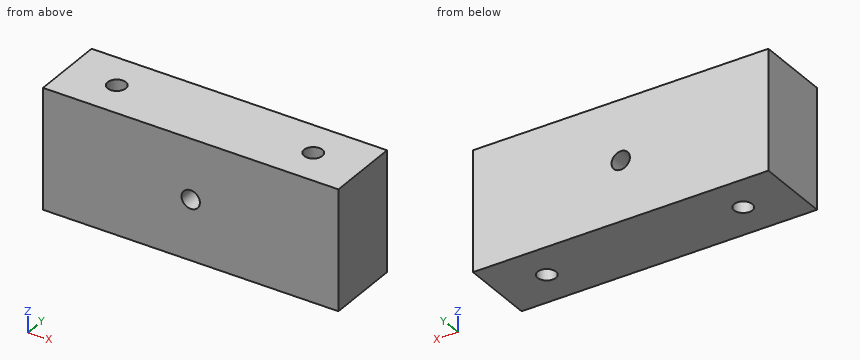
```python
from build123d import *

# Parameters (mm, degrees)
BOSS_EXTRUDE1_START     = 0.05
BOSS_EXTRUDE1_DEPTH     = 18.32
CUT_EXTRUDE1_DEPTH      = 168.935502816
CUT_EXTRUDE1_DEPTH_BACK = 168.935502816
SKETCH2_R               = 1.4
SKETCH3_R               = 1.4
CUT_EXTRUDE2_DEPTH      = 65.399803221


with BuildPart() as part:
    # Sketch1 → Boss-Extrude1 (new body)
    with BuildSketch(Plane.XY.offset(BOSS_EXTRUDE1_START)):
        Polygon((60.67170061, -154.017379901), (60.67170061, -144.167379901), (15.57170061, -144.167379901), (15.57170061, -154.017379901), (15.57170061, -155.517379901), (60.67170061, -155.517379901), align=None)
    extrude(amount=BOSS_EXTRUDE1_DEPTH)

    # Sketch2 → Cut-Extrude1 (cut, two sides: drawn at the far end of the back side and taken through both)
    with BuildSketch(Plane.XY.offset(18.37).offset(-CUT_EXTRUDE1_DEPTH_BACK)):
        with Locations((23.12170061, -149.842379901)):
            Circle(SKETCH2_R)
        with Locations((53.12170061, -149.842379901)):
            Circle(SKETCH2_R)
    extrude(amount=CUT_EXTRUDE1_DEPTH + CUT_EXTRUDE1_DEPTH_BACK, mode=Mode.SUBTRACT)

    # Sketch3 → Cut-Extrude2 (cut, through all)
    with BuildSketch(Plane(origin=(0, -144.167379901, 0), x_dir=(1, 0, 0), z_dir=(0, 1, 0))):
        with Locations(Location((38.12170061, -9.21, 0), (0, 0, 270))):
            Circle(SKETCH3_R)
    extrude(amount=-CUT_EXTRUDE2_DEPTH, mode=Mode.SUBTRACT)


solid = part.part
```
Could you check a few things on this model? Use its own coordinates, in mm. Coordinates: 2 decimals unless noted, no trailing zeros. Order: outer loops, then holes, each group sorted by start corner. A loop starts at its lowest first (then second) coordinate and runs counter-clockwise, first axis right, second up. Notation, with made-up numbers: M -16.75,28.5 L 4.25,28.5 A35 ccw 4.25,67.5 Z; hole C 14,12 d6. An arc over 180 degrees is marked long. Use one line per item in the form item = value. Start each with the question number.
1. Suppose I cut it at A-A on z = 9.21. Write out the boundary of the cut face in (x, y), then the cut area to 3 significant figures.
2. Suppose I cut it at C-C on z = 4.75. Write out the boundary of the cut face in (x, y), then the cut area to 3 significant figures.
3. Please list where these lines run through material, in increasing order: line 1 (X direction, y = -149.75, z = 5.5); line 2 (X direction, y = -150, z = 9.21); line 3 (X direction, y = -150.5, z = 6.25).
4. Suppose I cut it at B-B on y = -150.25. Write out the boundary of the cut face in (x, z).
Geometry says:
q1.outline = M 15.57,-155.52 L 36.72,-155.52 L 36.72,-144.17 L 15.57,-144.17 Z; M 39.52,-155.52 L 60.67,-155.52 L 60.67,-144.17 L 39.52,-144.17 Z; hole C 23.12,-149.84 d2.8; hole C 53.12,-149.84 d2.8
q1.area = 468 mm^2
q2.outline = M 15.57,-155.52 L 60.67,-155.52 L 60.67,-144.17 L 15.57,-144.17 Z; hole C 23.12,-149.84 d2.8; hole C 53.12,-149.84 d2.8
q2.area = 500 mm^2
q3.line_1 = 15.57 to 21.72, 24.52 to 51.72, 54.52 to 60.67
q3.line_2 = 15.57 to 21.73, 24.51 to 36.72, 39.52 to 51.73, 54.51 to 60.67
q3.line_3 = 15.57 to 21.89, 24.36 to 51.89, 54.36 to 60.67
q4.outline = M 15.57,0.05 L 21.78,0.05 L 21.78,18.37 L 15.57,18.37 Z; M 24.46,0.05 L 51.78,0.05 L 51.78,18.37 L 24.46,18.37 Z; M 54.46,0.05 L 60.67,0.05 L 60.67,18.37 L 54.46,18.37 Z; hole C 38.12,9.21 d2.8
